```python
from build123d import *

# Parameters (mm, degrees)
BOSS_EXTRUDE1_DEPTH = 4
SKETCH2_W           = 45
SKETCH2_H           = 4
BOSS_EXTRUDE2_DEPTH = 48
SKETCH3_R           = 1.25
CUT_EXTRUDE1_DEPTH  = 63.645625546
FILLET1_R           = 6
FILLET2_R           = 0.5
SKETCH6_R           = 2.255
CUT_EXTRUDE2_DEPTH  = 63.645625582
SKETCH7_R           = 1
CUT_EXTRUDE3_DEPTH  = 63.645625582
SKETCH8_R           = 4
CUT_EXTRUDE4_DEPTH  = 2.87
SKETCH9_R           = 3
CUT_EXTRUDE5_DEPTH  = 2.8
SKETCH10_R          = 2
SKETCH10_R_2        = 1.95
BOSS_EXTRUDE3_DEPTH = 3


with BuildPart() as part:
    # Sketch1 → Boss-Extrude1 (new body)
    with BuildSketch(Plane(origin=(0, 0, 0), x_dir=(1, 0, 0), z_dir=(0, 1, 0))):
        with BuildLine():
            Line((-22.5, -16.69), (22.5, -16.69))
            Line((22.5, -16.69), (22.5, 16.69))
            ThreePointArc((22.5, 16.69), (21.328427125, 19.518427125), (18.5, 20.69))
            Line((18.5, 20.69), (-18.5, 20.69))
            ThreePointArc((-18.5, 20.69), (-21.328427125, 19.518427125), (-22.5, 16.69))
            Line((-22.5, 16.69), (-22.5, -16.69))
        make_face()
    extrude(amount=BOSS_EXTRUDE1_DEPTH)

    # Sketch2 → Boss-Extrude2 (add)
    with BuildSketch(Plane.XZ):
        with Locations((0, 14.69)):
            Rectangle(SKETCH2_W, SKETCH2_H)
    extrude(amount=BOSS_EXTRUDE2_DEPTH)

    # Sketch3 → Cut-Extrude1 (cut, through all)
    with BuildSketch(Plane(origin=(0, 0, 12.69), x_dir=(-1, 0, 0), z_dir=(0, 0, -1))):
        with Locations((0, -39.35)):
            Circle(SKETCH3_R)
        with Locations((0, -24)):
            Circle(SKETCH3_R)
    extrude(amount=-CUT_EXTRUDE1_DEPTH, mode=Mode.SUBTRACT)

    # Fillet1
    fillet1_edges = [part.edges().sort_by_distance(p)[0] for p in [
        (-22.5, -48, 14.69),
        (22.5, -48, 14.69),
    ]]
    fillet(fillet1_edges, radius=FILLET1_R)

    # Fillet2
    fillet2_edges = [part.edges().sort_by_distance(p)[0] for p in [
        (22.5, -19, 16.69),
        (-22.5, -19, 16.69),
        (22.5, 4, 0),
        (21.328427125, 4, -19.518427125),
        (0, 4, -20.69),
        (-21.328427125, 4, -19.518427125),
        (0, -48, 16.69),
        (-20.742640687, -46.242640687, 16.69),
        (20.742640687, -46.242640687, 16.69),
        (-22.5, 4, 0),
        (0, 4, 16.69),
    ]]
    fillet(fillet2_edges, radius=FILLET2_R)

    # Sketch6 → Cut-Extrude2 (cut, through all)
    with BuildSketch(Plane(origin=(0, 0, 12.69), x_dir=(-1, 0, 0), z_dir=(0, 0, -1))):
        with Locations((0, -11)):
            Circle(SKETCH6_R)
    extrude(amount=-CUT_EXTRUDE2_DEPTH, mode=Mode.SUBTRACT)

    # Sketch7 → Cut-Extrude3 (cut, through all)
    with BuildSketch(Plane(origin=(0, 0, 12.69), x_dir=(-1, 0, 0), z_dir=(0, 0, -1))):
        with Locations((0, -19)):
            Circle(SKETCH7_R)
        with Locations((-5.656854249, -16.656854249)):
            Circle(SKETCH7_R)
        with Locations((-8, -11)):
            Circle(SKETCH7_R)
        with Locations((-5.656854249, -5.343145751)):
            Circle(SKETCH7_R)
        with Locations((0, -3)):
            Circle(SKETCH7_R)
        with Locations((5.656854249, -5.343145751)):
            Circle(SKETCH7_R)
        with Locations((8, -11)):
            Circle(SKETCH7_R)
        with Locations((5.656854249, -16.656854249)):
            Circle(SKETCH7_R)
    extrude(amount=-CUT_EXTRUDE3_DEPTH, mode=Mode.SUBTRACT)

    # Sketch8 → Cut-Extrude4 (cut)
    with BuildSketch(Plane.XY.offset(16.69)):
        with Locations((0, -11)):
            Circle(SKETCH8_R)
    extrude(amount=-CUT_EXTRUDE4_DEPTH, mode=Mode.SUBTRACT)

    # Sketch9 → Cut-Extrude5 (cut)
    with BuildSketch(Plane.XY.offset(16.69)):
        with Locations((0, -24)):
            Circle(SKETCH9_R)
        with Locations((0, -39.35)):
            Circle(SKETCH9_R)
    extrude(amount=-CUT_EXTRUDE5_DEPTH, mode=Mode.SUBTRACT)

    # Sketch10 → Boss-Extrude3 (add)
    with BuildSketch(Plane.XZ):
        with Locations(Location((16.5, -16.17, 0), (0, 0, 90))):
            Circle(SKETCH10_R)
        with Locations(Location((16.5, -4.17, 0), (0, 0, 90))):
            Circle(SKETCH10_R_2)
    extrude(amount=BOSS_EXTRUDE3_DEPTH)


solid = part.part
```
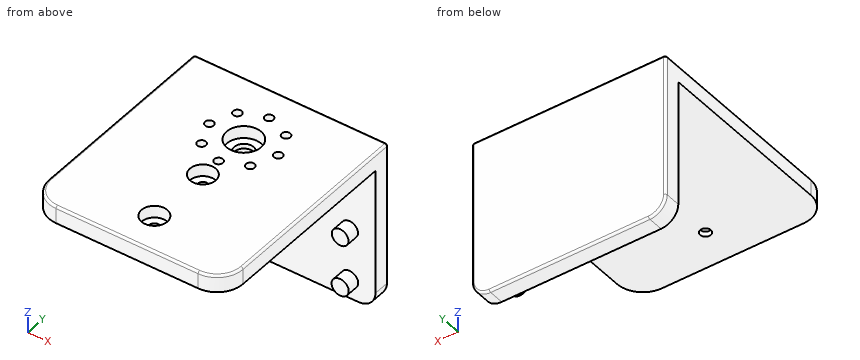
CAD build for the part. Positions are in the model's coordinates, mm. Coordinates: 2 decimals unless noted, no trailing zeros. Order: outer loops, then holes, each group sorted by start corner. A loop starts at its lowest first (then second) coordinate and runs counter-clockwise, first axis right, second up. Notation, with made-up numbers: M 88,44.5 L 125,44.5 A13 cw 125,52.5 Z; hole C -39.75,22 d5. An arc over 180 degrees is marked long. Answer as CSV lines item,"result".
1) Cut at D-D (x = -14). List the corners of the cut face in (y, z).
Verdict:
outline,"M -48,12.69 L 0,12.69 L 0,-20.69 L 3.5,-20.69 A0.5 ccw 4,-20.19 L 4,16.19 A0.5 ccw 3.5,16.69 L -47.5,16.69 A0.5 ccw -48,16.19 Z"
2) Drill centre lines: L1, parallel to Y at x = 0, z = 13.3 (3 decimals); L2, parallel to Y at x = 0, z = 14.9; L3, parallel to Y at x = 17.5, z = -0.5. Where is each one in solid material? Low to high. Write a range as from..to.
Verdict:
L1,"-48..-40.6, -38.1..-25.25, -22.75..-20, -18..-13.255, -8.745..-4, -2..4"
L2,"-48..-42.35, -36.35..-27, -21..-20, -18..-15, -7..-4, -2..4"
L3,"0..4"
3) Cut at A-A (y = -39.35). List the corners of the cut face in (x, z).
Verdict:
outline,"M -22.5,12.69 L -1.25,12.69 L -1.25,13.89 L -3,13.89 L -3,16.69 L -22,16.69 A0.5 ccw -22.5,16.19 Z; M 1.25,12.69 L 22.5,12.69 L 22.5,16.19 A0.5 ccw 22,16.69 L 3,16.69 L 3,13.89 L 1.25,13.89 Z"
4) Cut at B-B (x = -8). List the corners of the cut face in (y, z), then the cut area to 3 significant figures.
Verdict:
outline,"M -48,12.69 L -12,12.69 L -12,16.69 L -47.5,16.69 A0.5 ccw -48,16.19 Z; M -10,12.69 L 0,12.69 L 0,-20.69 L 3.5,-20.69 A0.5 ccw 4,-20.19 L 4,16.19 A0.5 ccw 3.5,16.69 L -10,16.69 Z"
area,"333 mm2"
5) Flat gauge pins, fed straight in: P1, Ø2.5, axis at x = 0, y = -3, coming from the -Z side; P2, Ø1.9, axis at x = 17, z = -4, coming from the -Y side; P3, Ø1.8, axis at x = 1, y = -39.5, coming from the +Z side. Where does each tip first touch, or does it go through?
Verdict:
P1,"z = 12.69"
P2,"y = -3"
P3,"z = 13.89"
6) Cut at C-C (y = -11). List the corners of the cut face in (x, z) (3 decimals), then the cut area to 3 significant figures.
Verdict:
outline,"M -22.5,12.69 L -9,12.69 L -9,16.69 L -22,16.69 A0.5 ccw -22.5,16.19 Z; M -7,12.69 L -2.255,12.69 L -2.255,13.82 L -4,13.82 L -4,16.69 L -7,16.69 Z; M 2.255,12.69 L 7,12.69 L 7,16.69 L 4,16.69 L 4,13.82 L 2.255,13.82 Z; M 9,12.69 L 22.5,12.69 L 22.5,16.19 A0.5 ccw 22,16.69 L 9,16.69 Z"
area,"136 mm2"
